The model under review builds one solid part; all positions refer to its coordinate system, in mm. Face numbers are marked on the shaded views. Round coordinates to 2 decimals unless told otherwise and drop trailing zeros. Loops run counter-clockwise (first coordinate to the right, second up) from the corner with the lowest first, then second, coordinate; pieces in that order, holes last. Notation, with made-up numbers: M 39.5,63.5 L 51.5,63.5 A21 cw 51.5,80.5 Z; hole C 2,71 d8. An arc over 180 degrees is marked long. Answer in a Markdown table with one row per item. Add a question column.
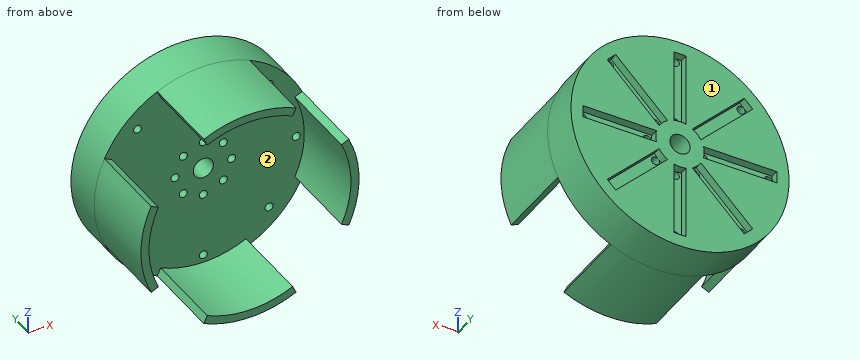
from build123d import *

# Parameters (mm, degrees)
SKETCH_1_R               = 27
EXTRUDE_1_DEPTH          = 10
SKETCH_2_R               = 2.5
CUT_EXTRUDE_1_DEPTH      = 15
EXTRUDE_2_DEPTH          = 20
CUT_EXTRUDE_2_DEPTH      = 2
SKETCH_5_R               = 1
CUT_EXTRUDE_3_DEPTH      = 37
CUT_EXTRUDE_3_DEPTH_BACK = 37


with BuildPart() as part:
    # Sketch 1 → Extrude 1 (new body)
    with BuildSketch(Plane(origin=(0, 0, 0), x_dir=(1, 0, 0), z_dir=(0, 1, 0))):
        Circle(SKETCH_1_R)
    extrude(amount=EXTRUDE_1_DEPTH)

    # Sketch 2 → Cut-Extrude 1 (cut)
    with BuildSketch(Plane(origin=(0, 10, 0), x_dir=(1, 0, 0), z_dir=(0, 1, 0))):
        Circle(SKETCH_2_R)
    extrude(amount=-CUT_EXTRUDE_1_DEPTH, mode=Mode.SUBTRACT)

    # Sketch 3 → Extrude 2 (add)
    with BuildSketch(Plane.XZ):
        with BuildLine():
            Line((-11.410693066, 24.47031025), (-10.565456543, 22.657694676))
            ThreePointArc((-10.565456543, 22.657694676), (1e-09, 25), (10.565456544, 22.657694676))
            Line((10.565456544, 22.657694676), (11.410693067, 24.47031025))
            ThreePointArc((11.410693067, 24.47031025), (1e-09, 27), (-11.410693066, 24.47031025))
        make_face()
        with BuildLine():
            Line((24.47031025, 11.410693066), (22.657694676, 10.565456543))
            ThreePointArc((22.657694676, 10.565456543), (25, -1e-09), (22.657694676, -10.565456544))
            Line((22.657694676, -10.565456544), (24.47031025, -11.410693067))
            ThreePointArc((24.47031025, -11.410693067), (27, -1e-09), (24.47031025, 11.410693066))
        make_face()
        with BuildLine():
            Line((11.410693066, -24.47031025), (10.565456543, -22.657694676))
            ThreePointArc((10.565456543, -22.657694676), (-1e-09, -25), (-10.565456544, -22.657694676))
            Line((-10.565456544, -22.657694676), (-11.410693067, -24.47031025))
            ThreePointArc((-11.410693067, -24.47031025), (-1e-09, -27), (11.410693066, -24.47031025))
        make_face()
        with BuildLine():
            Line((-24.47031025, -11.410693066), (-22.657694676, -10.565456543))
            ThreePointArc((-22.657694676, -10.565456543), (-25, 1e-09), (-22.657694676, 10.565456544))
            Line((-22.657694676, 10.565456544), (-24.47031025, 11.410693067))
            ThreePointArc((-24.47031025, 11.410693067), (-27, 1e-09), (-24.47031025, -11.410693066))
        make_face()
    extrude(amount=EXTRUDE_2_DEPTH)

    # Sketch 4 → Cut-Extrude 2 (cut)
    with BuildSketch(Plane(origin=(0, 10, 0), x_dir=(1, 0, 0), z_dir=(0, 1, 0))):
        with BuildLine():
            Line((-17.988048884, 15.888048884), (-5.160656882, 3.060656882))
            ThreePointArc((-5.160656882, 3.060656882), (-4.242640687, 4.242640687), (-3.060656882, 5.160656882))
            Line((-3.060656882, 5.160656882), (-15.888048884, 17.988048884))
            ThreePointArc((-15.888048884, 17.988048884), (-16.970562748, 16.970562748), (-17.988048884, 15.888048884))
        make_face()
        with BuildLine():
            Line((1.48492424, 23.954018452), (1.48492424, 5.813346713))
            ThreePointArc((1.48492424, 5.813346713), (0, 6), (-1.484924241, 5.813346713))
            Line((-1.484924241, 5.813346713), (-1.484924241, 23.954018452))
            ThreePointArc((-1.484924241, 23.954018452), (0, 24), (1.48492424, 23.954018452))
        make_face()
        with BuildLine():
            Line((17.988048884, 15.888048884), (5.160656882, 3.060656882))
            ThreePointArc((5.160656882, 3.060656882), (4.242640687, 4.242640687), (3.060656882, 5.160656882))
            Line((3.060656882, 5.160656882), (15.888048884, 17.988048884))
            ThreePointArc((15.888048884, 17.988048884), (16.970562748, 16.970562748), (17.988048884, 15.888048884))
        make_face()
        with BuildLine():
            Line((23.954018452, -1.48492424), (5.813346713, -1.48492424))
            ThreePointArc((5.813346713, -1.48492424), (6, 0), (5.813346713, 1.484924241))
            Line((5.813346713, 1.484924241), (23.954018452, 1.484924241))
            ThreePointArc((23.954018452, 1.484924241), (24, 0), (23.954018452, -1.48492424))
        make_face()
        with BuildLine():
            Line((15.888048884, -17.988048884), (3.060656882, -5.160656882))
            ThreePointArc((3.060656882, -5.160656882), (4.242640687, -4.242640687), (5.160656882, -3.060656882))
            Line((5.160656882, -3.060656882), (17.988048884, -15.888048884))
            ThreePointArc((17.988048884, -15.888048884), (16.970562748, -16.970562748), (15.888048884, -17.988048884))
        make_face()
        with BuildLine():
            Line((-1.48492424, -23.954018452), (-1.48492424, -5.813346713))
            ThreePointArc((-1.48492424, -5.813346713), (0, -6), (1.484924241, -5.813346713))
            Line((1.484924241, -5.813346713), (1.484924241, -23.954018452))
            ThreePointArc((1.484924241, -23.954018452), (0, -24), (-1.48492424, -23.954018452))
        make_face()
        with BuildLine():
            Line((-17.988048884, -15.888048884), (-5.160656882, -3.060656882))
            ThreePointArc((-5.160656882, -3.060656882), (-4.242640687, -4.242640687), (-3.060656882, -5.160656882))
            Line((-3.060656882, -5.160656882), (-15.888048884, -17.988048884))
            ThreePointArc((-15.888048884, -17.988048884), (-16.970562748, -16.970562748), (-17.988048884, -15.888048884))
        make_face()
        with BuildLine():
            Line((-23.954018452, 1.48492424), (-5.813346713, 1.48492424))
            ThreePointArc((-5.813346713, 1.48492424), (-6, 0), (-5.813346713, -1.484924241))
            Line((-5.813346713, -1.484924241), (-23.954018452, -1.484924241))
            ThreePointArc((-23.954018452, -1.484924241), (-24, 0), (-23.954018452, 1.48492424))
        make_face()
    extrude(amount=-CUT_EXTRUDE_2_DEPTH, mode=Mode.SUBTRACT)

    # Sketch 5 → Cut-Extrude 3 (cut, two sides)
    with BuildSketch(Plane(origin=(0, 10, 0), x_dir=(1, 0, 0), z_dir=(0, 1, 0))) as cut_extrude_3_sk:
        with Locations((-7, 0)):
            Circle(SKETCH_5_R)
        with Locations((-23, 0)):
            Circle(SKETCH_5_R)
        with Locations((-16.263455967, 16.263455967)):
            Circle(SKETCH_5_R)
        with Locations((-4.949747468, 4.949747468)):
            Circle(SKETCH_5_R)
        with Locations((0, 23)):
            Circle(SKETCH_5_R)
        with Locations((0, 7)):
            Circle(SKETCH_5_R)
        with Locations((16.263455967, 16.263455967)):
            Circle(SKETCH_5_R)
        with Locations((4.949747468, 4.949747468)):
            Circle(SKETCH_5_R)
        with Locations((23, 0)):
            Circle(SKETCH_5_R)
        with Locations((7, 0)):
            Circle(SKETCH_5_R)
        with Locations((16.263455967, -16.263455967)):
            Circle(SKETCH_5_R)
        with Locations((4.949747468, -4.949747468)):
            Circle(SKETCH_5_R)
        with Locations((0, -23)):
            Circle(SKETCH_5_R)
        with Locations((0, -7)):
            Circle(SKETCH_5_R)
        with Locations((-16.263455967, -16.263455967)):
            Circle(SKETCH_5_R)
        with Locations((-4.949747468, -4.949747468)):
            Circle(SKETCH_5_R)
    extrude(amount=CUT_EXTRUDE_3_DEPTH, mode=Mode.SUBTRACT)
    extrude(cut_extrude_3_sk.sketch, amount=-CUT_EXTRUDE_3_DEPTH_BACK, mode=Mode.SUBTRACT)


solid = part.part
1. Mouldability with a two-part tool opening along Z and no side actions: class the marked faces 1 and 2 as released by +Z, released by -Z, zero draft, split by the parting line, or undercut.
2. For pin 1 Ø2.5 at (x, z) = (-4.95, 4.95) entering from -Y; pin 2 Ø2.5 at (x, z) = (-14, 0.5) entering from +Y; pin 3 Ø1 at (y, z) = (9, -17) entering from +X; pin 4 Ø1.6 at (x, z) = (0, 23) entering from -Y, all flat-tipped, find the tip position at first contact; note any pin that passes through.
3. Take a section at C-C, the plane z = -7. State the section outline as (x, y) points, and give its area (3 significant figures).
4. To check wall thickness, follow probe 1 along Z at (x, y) = (0, 3); probe 2 along X at (y, z) = (3.5, 7). State the ranges of each line that lie inside material, in increasing order.
5. Take a section at A-A, the plane y = -16.25. State the section outline as (x, z) points, and give its area (3 significant figures).
6. Take a section at B-B, the plane x = 7. State the section outline as (y, z) points.
7. Take a section at D-D, the plane y = 6.5. State how many separate pieces and enclosed holes the cut face has, and give its area (3 significant figures).
Check sheet entries:
| question | item | result |
|---|---|---|
| 1 | face 1 | zero draft |
| 1 | face 2 | undercut |
| 2 | pin 1 | stops at y = 0 |
| 2 | pin 2 | stops at y = 10 |
| 2 | pin 3 | stops at x = 21.37 |
| 2 | pin 4 | passes through |
| 3 | outline | M -26.08,-20 L -24,-20 L -24,0 L -1,0 L -1,8 L -1.48,8 L -1.48,10 L -4.9,10 L -4.9,8 L -9.1,8 L -9.1,10 L -26.08,10 Z; M 1,0 L 24,0 L 24,-20 L 26.08,-20 L 26.08,10 L 9.1,10 L 9.1,8 L 4.9,8 L 4.9,10 L 1.48,10 L 1.48,8 L 1,8 Z |
| 3 | area | 566 mm^2 |
| 4 | probe 1 | z = -27 to -24, -22 to -8, -6 to -2.5, 2.5 to 6, 8 to 22, 24 to 27 |
| 4 | probe 2 | x = -26.08 to -1, 1 to 26.08 |
| 5 | outline | M -24.47,-11.41 L -22.66,-10.57 A25 cw -22.66,10.57 L -24.47,11.41 A27 ccw Z; M -11.41,-24.47 A27 ccw 11.41,-24.47 L 10.57,-22.66 A25 cw -10.57,-22.66 Z; M -11.41,24.47 L -10.57,22.66 A25 cw 10.57,22.66 L 11.41,24.47 A27 ccw Z; M 22.66,-10.57 L 24.47,-11.41 A27 ccw 24.47,11.41 L 22.66,10.57 A25 cw Z |
| 5 | area | 182 mm^2 |
| 6 | outline | M -20,-26.08 L 10,-26.08 L 10,-9.1 L 8,-9.1 L 8,-4.9 L 10,-4.9 L 10,-1.48 L 8,-1.48 L 8,-1 L 0,-1 L 0,-24 L -20,-24 Z; M -20,24 L 0,24 L 0,1 L 8,1 L 8,1.48 L 10,1.48 L 10,4.9 L 8,4.9 L 8,9.1 L 10,9.1 L 10,26.08 L -20,26.08 Z |
| 7 | separate pieces | 1 |
| 7 | enclosed holes | 17 |
| 7 | area | 2,220 mm^2 |
